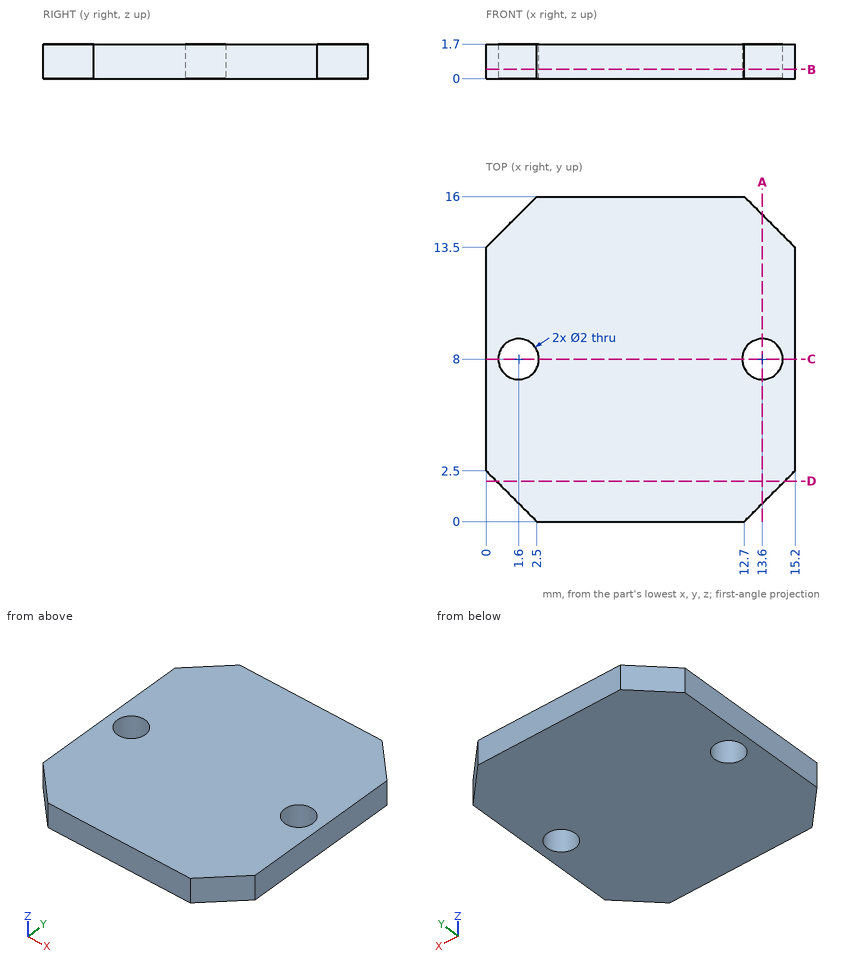
Geometry check sheet. Reference: drawing and pictorial views, mm from the part's lowest x, y, z. Round coordinates to 2 decimals unless told otherwise and drop trailing zeros. Order: outer loops, then holes, each group sorted by start corner. A loop starts at its lowest first (then second) coordinate and runs counter-clockwise, first axis right, second up. Notation, with made-up numbers: (47, 77.5) - (61, 77.5) arc R21 cw to (61, 111.5) - close; hole circle Ø7 at (-31, 15). An arc over 180 degrees is marked (long way). Use a Markdown table: item, result. Add a question column.
1) Section check A-A (x = 13.6). Record the cut outline in (y, z), then the cut area to 3 significant figures.
2) Section check B-B (z = 0.45). Record the cut outline in (x, y), then the cut area to 3 significant figures.
3) Thickness scan on line 1 along Y through (x, z) = (13.6, 0.95); line 2 along Y through (x, z) = (14.75, 1.25); line 3 along X through (y, z) = (2, 1.5). Record the ranges inside material, lowest first.
4) Section check D-D (y = 2). Record the cut outline in (x, z).
5) Gauge pin test, flat end, axial feed: P1, Ø1.2, axis at x = 13.6, y = 8, coming from the -Z side. Record the tip position at first contact, or that the pin passes through.
6) Section check C-C (y = 8). Record the cut outline in (x, z).
Established:
| question | item | result |
|---|---|---|
| 1 | outline | (0.9, 0) - (7, 0) - (7, 1.7) - (0.9, 1.7) - close; (9, 0) - (15.1, 0) - (15.1, 1.7) - (9, 1.7) - close |
| 1 | area | 20.7 mm2 |
| 2 | outline | (0, 2.5) - (2.5, 0) - (12.7, 0) - (15.2, 2.5) - (15.2, 13.5) - (12.7, 16) - (2.5, 16) - (0, 13.5) - close; hole circle Ø2 at (1.6, 8); hole circle Ø2 at (13.6, 8) |
| 2 | area | 224 mm2 |
| 3 | line 1 | 0.9 to 7, 9 to 15.1 |
| 3 | line 2 | 2.05 to 13.95 |
| 3 | line 3 | 0.5 to 14.7 |
| 4 | outline | (0.5, 0) - (14.7, 0) - (14.7, 1.7) - (0.5, 1.7) - close |
| 5 | P1 | through |
| 6 | outline | (0, 0) - (0.6, 0) - (0.6, 1.7) - (0, 1.7) - close; (2.6, 0) - (12.6, 0) - (12.6, 1.7) - (2.6, 1.7) - close; (14.6, 0) - (15.2, 0) - (15.2, 1.7) - (14.6, 1.7) - close |
